```python
from build123d import *

# Parameters (mm, degrees)
F1_DEPTH      = 16
F1_DEPTH_BACK = 16
F3_DEPTH      = 55
F8_R          = 1.75
F9_DEPTH      = 25
F10_R         = 3.05
F11_DEPTH     = 3.5


with BuildPart() as f1:
    # F0 (on Front) → F1 (new body, two sides)
    with BuildSketch(Plane.XZ) as f1_sk:
        with BuildLine():
            ThreePointArc((8.5, -14.25), (0, 0), (8.5, 14.25))
            Line((8.5, 14.25), (20.5, 14.25))
            ThreePointArc((20.5, 14.25), (18.1568542495, 19.9068542495), (12.5, 22.25))
            Line((12.5, 22.25), (2.3706777177, 22.25))
            ThreePointArc((2.3706777177, 22.25), (-6.6993882302, 12.7288664774), (-10, 0))
            Line((-10, 0), (-10, -22.25))
            Line((-10, -22.25), (25.5, -22.25))
            ThreePointArc((25.5, -22.25), (31.1568542495, -19.9068542495), (33.5, -14.25))
            Line((33.5, -14.25), (8.5, -14.25))
        make_face()
    extrude(amount=F1_DEPTH)
    extrude(f1_sk.sketch, amount=-F1_DEPTH_BACK)

    # F2 (on face) → F3 (join)
    with BuildSketch(Plane(origin=(-10, 0, 0), x_dir=(0, -1, 0), z_dir=(-1, 0, 0))):
        with BuildLine():
            Line((16, -9.75), (16, -4.75))
            ThreePointArc((16, -4.75), (0, -0.8787648325), (-16, -4.75))
            Line((-16, -4.75), (-16, -9.75))
            ThreePointArc((-16, -9.75), (0, -13.6212351675), (16, -9.75))
        make_face()
    extrude(amount=F3_DEPTH)

    # F3_face (on face) → F5 section 0
    with BuildSketch(Plane(origin=(-10, 0, -17.2392152615), x_dir=(0, -1, 0), z_dir=(-1, 0, 0))):
        with BuildLine():
            ThreePointArc((16, 7.4892152615), (0, 3.617980094), (-16, 7.4892152615))
            Line((-16, 7.4892152615), (-16, -5.0107847385))
            Line((-16, -5.0107847385), (16, -5.0107847385))
            Line((16, -5.0107847385), (16, 7.4892152615))
        make_face()
    # F3_face1 (on face) → F5 section 1
    with BuildSketch(Plane(origin=(-65, 0, -7.25), x_dir=(0, -1, 0), z_dir=(-1, 0, 0))):
        with BuildLine():
            Line((-16, 2.5), (-16, -2.5))
            ThreePointArc((-16, -2.5), (0, -6.3712351675), (16, -2.5))
            Line((16, -2.5), (16, 2.5))
            ThreePointArc((16, 2.5), (0, 6.3712351675), (-16, 2.5))
        make_face()
    loft()

    # F3_face1 (on face) → F7 section 0
    with BuildSketch(Plane(origin=(-65, 0, -7.25), x_dir=(0, -1, 0), z_dir=(-1, 0, 0))):
        with BuildLine():
            Line((-16, 2.5), (-16, -2.5))
            ThreePointArc((-16, -2.5), (0, -6.3712351675), (16, -2.5))
            Line((16, -2.5), (16, 2.5))
            ThreePointArc((16, 2.5), (0, 6.3712351675), (-16, 2.5))
        make_face()
    # F6 (on offset) → F7 section 1
    with BuildSketch(Plane(origin=(-75, 0, 0), x_dir=(0, -1, 0), z_dir=(-1, 0, 0))):
        with BuildLine():
            ThreePointArc((-16, -1.75), (0, -5.6212351675), (16, -1.75))
            Line((16, -1.75), (16, 3.25))
            ThreePointArc((16, 3.25), (0, 7.1212351675), (-16, 3.25))
            Line((-16, 3.25), (-16, -1.75))
        make_face()
    loft()

    # F8 (on face) → F9 (cut)
    with BuildSketch(Plane(origin=(0, 0, -22.25), x_dir=(1, 0, 0), z_dir=(0, 0, -1))):
        with Locations((17.5, 0)):
            Circle(F8_R)
    extrude(amount=-F9_DEPTH, mode=Mode.SUBTRACT)

    # F10 (on face) → F11 (cut)
    with BuildSketch(Plane.XY.offset(-14.25)):
        with Locations((17.5, 0)):
            Circle(F10_R)
    extrude(amount=-F11_DEPTH, mode=Mode.SUBTRACT)


solid = f1.part
```
The listing builds one solid part. Answer for the finished solid, in the listing's coordinates (mm). A direction names the side the tool comes from. Give positions to 0.01 mm unless a question says otherwise; leave off trailing zeros. Loops run counter-clockwise (first coordinate to the right, second up) from the corner with the lowest first, then second, coordinate; pieces in that order, holes last. Notation, with made-up numbers: M 31,-11.5 L 72,-11.5 A6 cw 72,-4.5 Z; hole C 14.5,51.25 d8. An arc over 180 degrees is marked long. One line per item, written item: value.
1. For faces 4 (the face through (21, 0, -14.25)), 5 (the face through (-6.61, -0.22, 12.89)), 6 (the face through (-37.11, -0.23, -0.88)), 7 (the face through (17, -2, -17.75)), determine the directions among +Z, -Z, +X, -X, +Y, -Y from which every point of the face is accessible in a straight line to the end or side of a thin tool.
Found:
face 4: +X, +Y, -Y
face 5: +Z, +Y, -Y
face 6: +Z
face 7: none
2. Find the intervals of material crossed by probe 1 along Y at (x, z) = (17.5, -20.3); probe 2 along Y at (x, z) = (17.5, -16.5); probe 3 along Z at (x, y) = (17.5, -12.5) (3 decimals), in increasing order.
Found:
probe 1: -16 to -1.75, 1.75 to 16
probe 2: -16 to -3.05, 3.05 to 16
probe 3: -22.25 to -14.25, 14.25 to 20.495
3. Each of these flat-tipped pins is pushed along its axis until it touches: P1, Ø4, axis at x = -44.5, y = -6, coming from the +Z side; P2, Ø1, axis at y = -7, z = 9.5, coming from the +X side; P3, Ø2, axis at x = 17.5, y = 0, coming from the -Z side. Where does it stop, or does it pass through?
Found:
P1: z = -1.11
P2: x = 3.46
P3: z = 14.25
4. Section B-B on z = 16 is taken. Determine the outline of the cut face in (x, y), plus the area to 3 significant figures.
Found:
outline: M -4.55,-16 L 20.31,-16 L 20.31,16 L -4.55,16 Z
area: 795 mm^2
5. Section A-A on x = 17.5 is taken. Determine the outline of the cut face in (y, z) (3 decimals), plus the area to 3 significant figures.
Found:
outline: M -16,-22.25 L -1.75,-22.25 L -1.75,-17.75 L -3.05,-17.75 L -3.05,-14.25 L -16,-14.25 Z; M -16,14.25 L 16,14.25 L 16,20.495 L -16,20.495 Z; M 1.75,-22.25 L 16,-22.25 L 16,-14.25 L 3.05,-14.25 L 3.05,-17.75 L 1.75,-17.75 Z
area: 419 mm^2
6. For a pull along Y with two mould halves and no side action, classify faces 1 (the face through (8, 0, -22.25)), 2 (the face through (-13, 16, -9)), 3 (the face through (16.11, 1.06, -20.03)) as pulls with the +Y half, pulls with the -Y half, needs draft (parallel to the pull), parting line crosses it, or undercut.
Found:
face 1: needs draft
face 2: pulls with the +Y half
face 3: undercut
